Can you work these out from the drawing? Everything is in mm from the part's minimum corner. Give positions to 0.01 mm unless a question says otherwise; leave off trailing zeros. Order: outer loops, then holes, each group sorted by start corner. A loop starts at its lowest first (then second) coordinate and runs counter-clockwise, first axis right, second up. Notation, with made-up numbers: (3, 69) - (35, 69) arc R32 ccw to (35, 100) - close; hole circle Ø4 at (72.5, -15.75). An arc over 180 degrees is marked (long way). Answer as a JSON object with one key per item and string values.
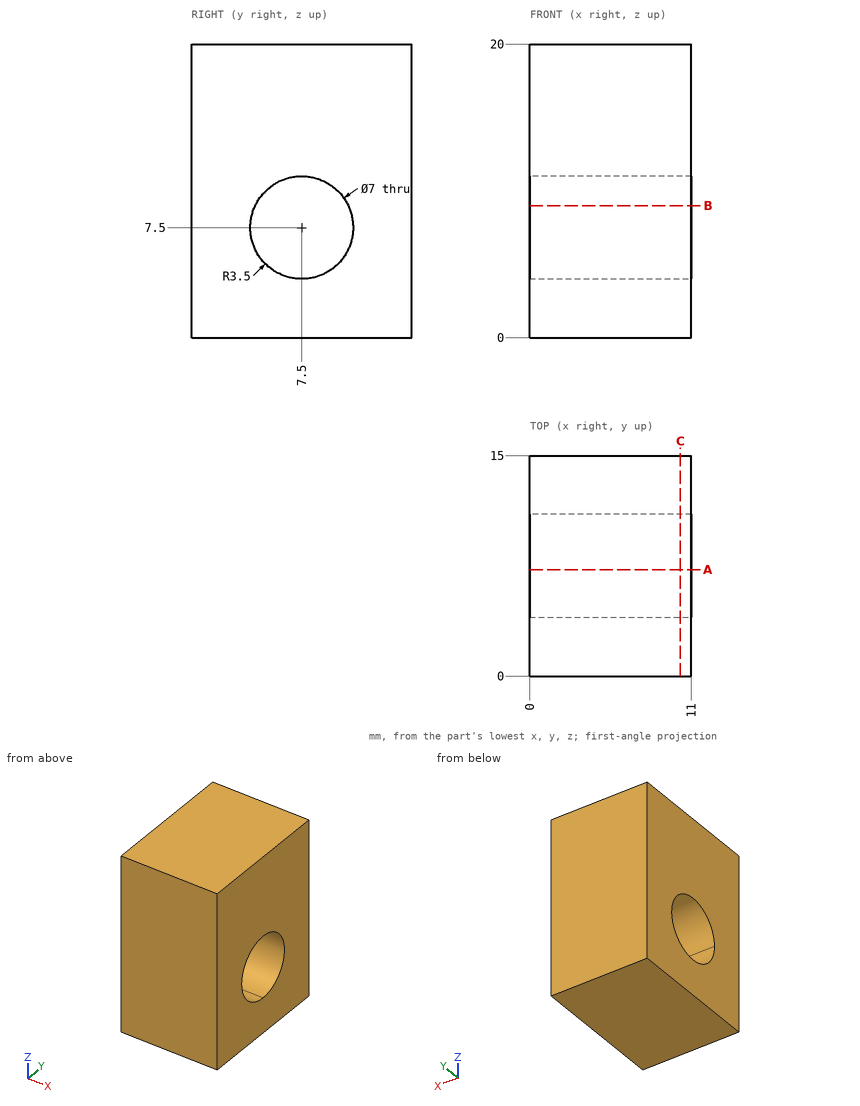
Q1. If we section it at C-C, the plane x = 10.25: Please give me the cut outline in (y, z).
Recorded:
{"outline": "(0, 0) - (15, 0) - (15, 20) - (0, 20) - close; hole circle Ø7 at (7.5, 7.5)"}
Q2. If we section it at B-B, the plane z = 9: Please give me the cut outline in (x, y).
Recorded:
{"outline": "(0, 0) - (11, 0) - (11, 4.34) - (0, 4.34) - close; (0, 10.66) - (11, 10.66) - (11, 15) - (0, 15) - close"}
Q3. I need wall thicknesses on L1, parallel to Z at x = 3.5, y = 7.5; L2, parallel to Y at x = 4.5, z = 7.5; L3, parallel to Y at x = 10.75, z = 9.25. Which ranges of each line are inside material? Lowest first, please.
Recorded:
{"L1": "z = 0 to 4, 11 to 20", "L2": "y = 0 to 4, 11 to 15", "L3": "y = 0 to 4.47, 10.53 to 15"}
Q4. If we section it at A-A, the plane y = 7.25: Please give me the cut outline in (x, z).
Recorded:
{"outline": "(0, 0) - (11, 0) - (11, 4.01) - (0, 4.01) - close; (0, 10.99) - (11, 10.99) - (11, 20) - (0, 20) - close"}
